Read the model definition and answer for the solid it produces. Units are mm, in the model's axes. A direction names the side the tool comes from. Coordinates: 2 decimals unless noted, no trailing zeros. Write each loop counter-clockwise with the first axis right and the second up, starting at its lowest first coordinate (ties: lowest second). Pieces come first, ordered by that corner, then holes.
1) Find the intervals of material crossed by line 1 (Z direction, x = 0, y = 6.5); line 2 (Z direction, x = 2, y = -5.25); line 3 (X direction, y = -3, z = -45), in increasing order.
2) The part is cut by section A-A (z = -54). Determine the outline of the cut face in (x, y), then the cut area to 3 significant figures.
3) Each of these flat-tipped pins is pushed along its axis until it touches: pin 1 Ø3 at (x, y) = (-3.5, -3.5) entering from -Z; pin 2 Ø8 at (y, z) = (3, -86) entering from +X; pin 3 Ø1.5 at (y, z) = (5, -66) entering from -X. Where does it stop, or does it pass through?
4) Which of the six approach directions +Z, -Z, +X, -X, +Y, -Y give full straight-line access (tool end or side, diameter ignored) to faces 1 (the face through (-1.08, -4.88, -25.21)), 2 (the face through (-1.08, -4.88, 9.86)), 3 (the face through (0.867, -3.905, -93.902))?
from build123d import *

# Parameters (mm, degrees)
SKETCH_1_R          = 7.5
EXTRUDE_1_DEPTH     = 51
SKETCH_2_R          = 5
EXTRUDE_2_DEPTH     = 20
EXTRUDE_START       = 36
SKETCH_3_R          = 5
EXTRUDE_3_DEPTH     = 36
SKETCH_4_OUTSIDE_W  = 38.816
SKETCH_4_OUTSIDE_H  = 38.816
SKETCH_4_OUTSIDE_R  = 5
CUT_EXTRUDE_1_DEPTH = 46
SKETCH_5_R          = 4
EXTRUDE_4_DEPTH     = 15
SKETCH_6_R          = 5
EXTRUDE_5_DEPTH     = 20
EXTRUDE_5_TAPER     = 2.8625
EXTRUDE_START_2     = 7.5
SKETCH_7_R          = 4
EXTRUDE_6_DEPTH     = 7.5
CHAMFER_1_SIZE      = 2.5
CHAMFER_2_SIZE      = 1


with BuildPart() as part:
    # Эскиз1 → Бобышка-Вытянуть1 (new body)
    with BuildSketch(Plane.XY):
        Circle(SKETCH_1_R)
    extrude(amount=-EXTRUDE_1_DEPTH)

    # Эскиз2 → Бобышка-Вытянуть2 (add)
    with BuildSketch(Plane.XY):
        Circle(SKETCH_2_R)
    extrude(amount=EXTRUDE_2_DEPTH)

    # Эскиз3 → Бобышка-Вытянуть3 (add)
    with BuildSketch(Plane(origin=(0, 0, -51), x_dir=(-1, 0, 0), z_dir=(0, 0, -1)).offset(EXTRUDE_START)):
        with Locations(Location((0, 0, 0), (0, 0, 180))):
            Circle(SKETCH_3_R)
    extrude(amount=-EXTRUDE_3_DEPTH)

    # Эскиз4 outside → Вырез-Вытянуть1 (cut)
    with BuildSketch(Plane.XY.offset(-2.5)):
        Rectangle(SKETCH_4_OUTSIDE_W, SKETCH_4_OUTSIDE_H)
        Circle(SKETCH_4_OUTSIDE_R, mode=Mode.SUBTRACT)
    extrude(amount=-CUT_EXTRUDE_1_DEPTH, mode=Mode.SUBTRACT)

    # Эскиз5 → Бобышка-Вытянуть4 (add)
    with BuildSketch(Plane(origin=(0, 0, -87), x_dir=(-1, 0, 0), z_dir=(0, 0, -1))):
        Circle(SKETCH_5_R)
    extrude(amount=EXTRUDE_4_DEPTH)

    # Эскиз6 → Бобышка-Вытянуть5 (add)
    with BuildSketch(Plane.XY.offset(20)):
        Circle(SKETCH_6_R)
    extrude(amount=EXTRUDE_5_DEPTH, taper=EXTRUDE_5_TAPER)

    # Эскиз7 → Бобышка-Вытянуть6 (add)
    with BuildSketch(Plane.XY.offset(40).offset(EXTRUDE_START_2)):
        with Locations(Location((0, 0, 0), (0, 0, 180))):
            Circle(SKETCH_7_R)
    extrude(amount=-EXTRUDE_6_DEPTH)

    # Фаска1
    chamfer_1_edges = [part.edges().sort_by_distance(p)[0] for p in [
        (-5, 0, -48.5),
        (-5, 0, -2.5),
    ]]
    chamfer(chamfer_1_edges, length=CHAMFER_1_SIZE - 0.0001)  # a hair under: the kernel refuses the full size

    # Фаска2
    chamfer_2_edges = [part.edges().sort_by_distance(p)[0] for p in [
        (4, 0, -102),
        (4, 0, 47.5),
    ]]
    chamfer(chamfer_2_edges, length=CHAMFER_2_SIZE)


solid = part.part
Reported:
1. line 1: z = -51 to -47.5, -3.5 to 0
1. line 2: z = -51 to -46.62, -4.38 to 0
1. line 3: x = -4 to 4
2. outline: circle Ø10 at (0, 0)
2. area: 78.5 mm2
3. pin 1: stops at z = -101.55
3. pin 2: stops at x = 5
3. pin 3: stops at x = -2.63
4. face 1: none
4. face 2: +Z
4. face 3: -Z
